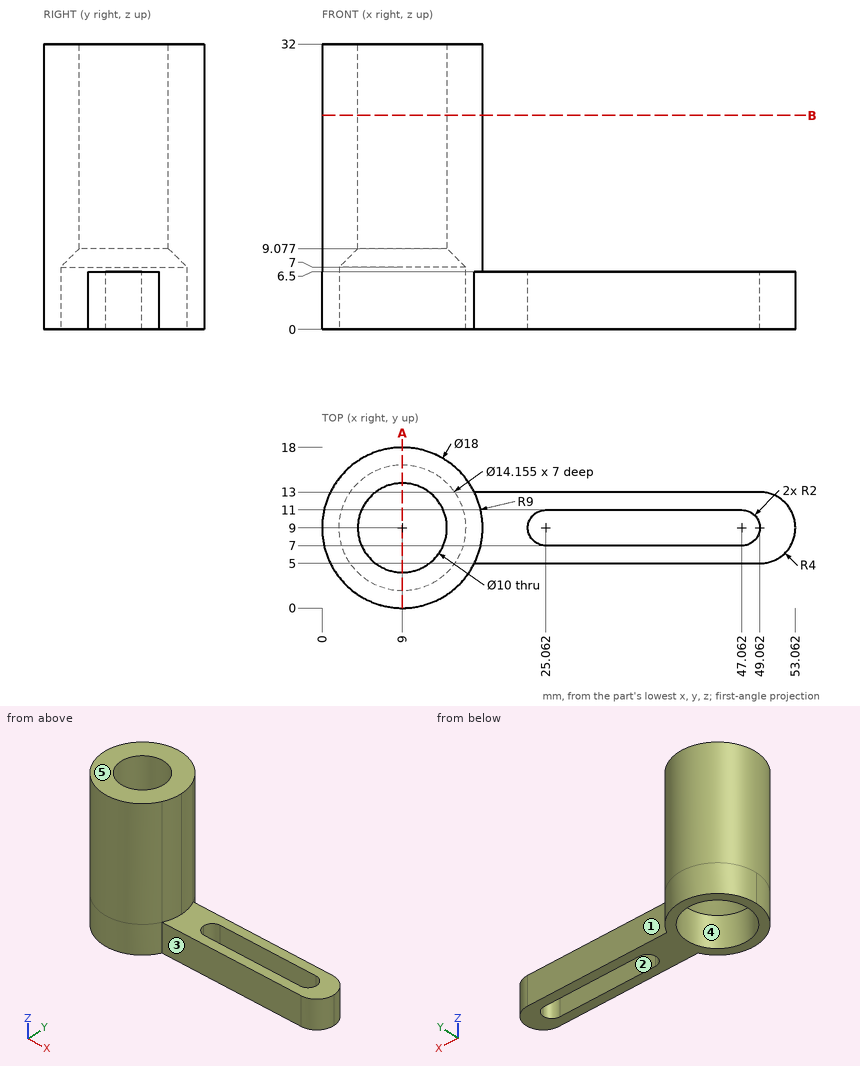
Drawing for the job (mm, zero at the part's lowest x, y, z). A direction names the side the tool comes from. Give positions to 0.01 mm unless a question says otherwise; leave off trailing zeros. Order: outer loops, then holes, each group sorted by start corner. A loop starts at its lowest first (then second) coordinate and runs counter-clockwise, first axis right, second up. Notation, with made-up numbers: (60.5, 6.5) - (66.5, 6.5) arc R25 cw to (66.5, 35.5) - close; hole circle Ø6 at (16, -34.5). An arc over 180 degrees is marked (long way). Use one line per item in the form item = value.
Item 1: Slice it at B-B on z = 24. Give the cut face in (x, y), and give its area (3 significant figures).
Solution:
outline = circle Ø18 at (9, 9); hole circle Ø10 at (9, 9)
area = 176 mm2
Item 2: Slice it at A-A on x = 9. Give the cut face in (y, z).
Solution:
outline = (0, 0) - (1.92, 0) - (1.92, 7) - (4, 9.08) - (4, 32) - (0, 32) - close; (14, 9.08) - (16.08, 7) - (16.08, 0) - (18, 0) - (18, 32) - (14, 32) - close
Item 3: Probe probe 1 along Y at (x, z) = (28, 6); probe 2 along Y at (x, z) = (9, 4.25); probe 3 along X at (y, z) = (5.5, 17). List the from-to ranges inside material, lowest first. Write a range as from..to.
Solution:
probe_1 = 5..7, 11..13
probe_2 = 0..1.92, 16.08..18
probe_3 = 0.71..5.43, 12.57..17.29
Item 4: Which spindle directions (+Z, -Z, +X, -X, +Y, -Y) get a long thin tool onto all of the face, cutting with end or side? Do the marked faces 4 and 5. Say none if no direction does.
Solution:
face_4 = -Z
face_5 = +Z, +X, -X, +Y, -Y
Item 5: Two-plate mould, pull along Y, no slides. Class the marked faces 1, 2 and 3: released by +Y, released by -Y, zero draft, split by the parting line, or undercut.
Solution:
face_1 = released by +Y
face_2 = undercut
face_3 = released by -Y
Item 6: Pin check, flat tips, straight feed: pin 1 Ø1 at (y, z) = (2, 9) entering from +X (1 decimal); pin 2 Ø5 at (x, z) = (27.5, 2) entering from +Y; pin 3 Ø2 at (x, z) = (37.5, 3) entering from -Y. Stop position of each tip, or through.
Solution:
pin_1 = 15.2
pin_2 = 13
pin_3 = 5
